Verification items for the finished model (mm, model axes). A direction names the side the tool comes from. Give positions to 0.01 mm unless a question says otherwise; leave off trailing zeros. Loops run counter-clockwise (first coordinate to the right, second up) from the corner with the lowest first, then second, coordinate; pieces in that order, holes last. Notation, with made-up numbers: (22, -9.75) - (49, -9.75) arc R32 cw to (49, 18.25) - close; hole circle Ø7 at (-12.5, 72). An arc over 180 degrees is marked (long way). One line per item, written item: value. Start each with the question number.
1. Gauge pin test, flat ends, axial feed: pin 1 (1 mm diameter, centred on x = -10, y = -7, fed in from -Z); pin 2 (12 mm diameter, centred on x = 0, y = 0, fed in from -Z). Record the tip position at first contact, or that the pin passes through.
2. Scan lines: L1, parallel to Y at x = 8.5, z = 31.5; L2, parallel to Y at x = 0, z = 44.2. Record each from-to range of solid material in increasing order. Write a range as [from, to].
3. Sectioned sample at B-B (x = -0.5). Record the cut outline in (y, z), plus the area to 3 significant figures.
4. Sectioned sample at D-D (x = -4.5). Record the cut outline in (y, z), plus the area to 3 significant figures.
5. Sectioned sample at C-C (z = 41.5). Record the cut outline in (x, y).
6. Access from +Z, -Z, +X, -X, +Y, -Y to the whole of each face (thin tool, end or side, straight path). Record for faces 5 (the cylindrical face through (13.246, 13.206, 23.369)), 6 (the cylindrical face through (-5.36, 8.406, 44.432)).
7. Sectioned sample at A-A (y = 0). Record the cut outline in (x, z) (1 decimal), plus the area to 3 significant figures.
8. Mould release check, pull along Y, two halves, no side actions. Record for faces 1 (the cylindrical face through (13.206, -13.246, 23.369)), 2 (the flat face through (0, 13.97, 26)), 3 (the flat face through (0, 16.51, 27)), 4 (the cylindrical face through (14.982, -15.061, 23.18)): pulls with the +Y half, pulls with the -Y half, needs draft (parallel to the pull), parting line crosses it, or undercut.
from build123d import *

# Parameters (mm, degrees)
F0_W     = 33.02
F0_H     = 33.02
F0_R     = 9.9695
F1_DEPTH = 45.72
F2_R     = 5.08
F3_T     = -2.54
F5_D     = 19.939
F7_DEPTH = 33.021


with BuildPart() as f1:
    # F0 (on Top) → F1 (new body)
    with BuildSketch(Plane.XY):
        Rectangle(F0_W, F0_H)
        Circle(F0_R, mode=Mode.SUBTRACT)
        Circle(F0_R)
    extrude(amount=F1_DEPTH)

    # F2
    f2_edges = [f1.edges().sort_by_distance(p)[0] for p in [
        (-16.51, -16.51, 22.86),
        (16.51, -16.51, 22.86),
        (16.51, 16.51, 22.86),
        (-16.51, 16.51, 22.86),
    ]]
    fillet(f2_edges, radius=F2_R)

    # F3
    f3_openings = [f1.faces().sort_by_distance(p)[0] for p in [
        (0, 0, 0),
    ]]
    offset(amount=F3_T, openings=f3_openings)

    # F5 (through all)
    with Locations(Plane.XY.offset(45.72)):
        with Locations((0, 0)):
            Hole(F5_D / 2)

    # F6 (on face) → F7 (cut, through all)
    with BuildSketch(Plane(origin=(0, 16.51, 0), x_dir=(-1, 0, 0), z_dir=(0, 1, 0))):
        with BuildLine():
            Line((11.43, 0), (14.2875, 0))
            ThreePointArc((14.2875, 0), (13.5543126209, 4.518104207), (11.43, 8.5725))
            Line((11.43, 8.5725), (11.43, 0))
        make_face()
        with BuildLine():
            Line((-11.43, 0), (-11.43, 8.5725))
            ThreePointArc((-11.43, 8.5725), (-13.5543126209, 4.518104207), (-14.2875, 0))
            Line((-14.2875, 0), (-11.43, 0))
        make_face()
        with BuildLine():
            Line((11.43, 0), (11.43, 8.5725))
            ThreePointArc((11.43, 8.5725), (0, 14.2875), (-11.43, 8.5725))
            Line((-11.43, 8.5725), (-11.43, 0))
            Line((-11.43, 0), (11.43, 0))
        make_face()
    extrude(amount=-F7_DEPTH, mode=Mode.SUBTRACT)


solid = f1.part
Results are:
1. pin 1: stops at z = 43.18
1. pin 2: passes through
2. L1: y = [-16.51, -13.97], [13.97, 16.51]
2. L2: y = [-16.51, -9.97], [9.97, 16.51]
3. outline: (-16.51, 14.28) - (-13.97, 14.28) - (-13.97, 43.18) - (-9.96, 43.18) - (-9.96, 45.72) - (-16.51, 45.72) - close; (9.96, 43.18) - (13.97, 43.18) - (13.97, 14.28) - (16.51, 14.28) - (16.51, 45.72) - (9.96, 45.72) - close
3. area: 180 mm^2
4. outline: (-16.51, 13.56) - (-13.97, 13.56) - (-13.97, 43.18) - (-8.9, 43.18) - (-8.9, 45.72) - (-16.51, 45.72) - close; (8.9, 43.18) - (13.97, 43.18) - (13.97, 13.56) - (16.51, 13.56) - (16.51, 45.72) - (8.9, 45.72) - close
4. area: 189 mm^2
5. outline: (-16.51, -11.43) arc R5.08 ccw to (-11.43, -16.51) - (11.43, -16.51) arc R5.08 ccw to (16.51, -11.43) - (16.51, 11.43) arc R5.08 ccw to (11.43, 16.51) - (-11.43, 16.51) arc R5.08 ccw to (-16.51, 11.43) - close; hole (-13.97, -11.43) arc R2.54 ccw to (-11.43, -13.97) - (11.43, -13.97) arc R2.54 ccw to (13.97, -11.43) - (13.97, 11.43) arc R2.54 ccw to (11.43, 13.97) - (-11.43, 13.97) arc R2.54 ccw to (-13.97, 11.43) - close
6. face 5: -Z
6. face 6: +Z, -Z
7. outline: (-16.5, 0) - (-14.3, 0) arc R14.3 cw to (-14, 3) - (-14, 43.2) - (-10, 43.2) - (-10, 45.7) - (-16.5, 45.7) - close; (10, 43.2) - (14, 43.2) - (14, 3) arc R14.3 cw to (14.3, 0) - (16.5, 0) - (16.5, 45.7) - (10, 45.7) - close
7. area: 251 mm^2
8. face 1: undercut
8. face 2: undercut
8. face 3: pulls with the +Y half
8. face 4: pulls with the -Y half
